CAD build for the part. Positions are in the model's coordinates, mm. A direction names the side the tool comes from. Give positions to 0.01 mm unless a question says otherwise; leave off trailing zeros. Order: outer loops, then holes, each group sorted by start corner. A loop starts at its lowest first (then second) coordinate and runs counter-clockwise, first axis right, second up. Notation, with made-up numbers: M -15.75,-7.5 L -10.75,-7.5 A13 cw -10.75,12.5 Z; hole C -1,71 d9. An arc over 180 degrees is marked long. Put each result on its own line as item: value. Start each with the question number.
1) Two-plate mould, pull along X, no slides. Class faces 1 (the face through (-26.03, 0.14, 1.61)), 2 (the face through (-0.296, 0.078, 15.872)), 3 (the face through (-19, 0, 0)): released by +X, released by -X, zero draft, split by the parting line, or undercut.
2) Cut at A-A (y = 0). Write the cut outline in (x, z) (3 decimals).
3) Drill centre lines: line 1 (Y direction, x = -22.86, z = 2.05) (3 decimals); line 2 (Z direction, x = 17.5, y = 2.5) (3 decimals); line 3 (X direction, y = -2.25, z = 9.5). Where is each one in solid material? Low to high. Write a range as [from, to].
4) Cut at C-C (z = 1.5). Write the cut outline in (x, y) (3 decimals), and give its area (3 significant figures).
5) Cut at B-B (x = -22.86). Write the cut outline in (y, z) (3 decimals).
6) Pin check, flat tips, straight feed: pin 1 (2 mm diameter, centred on y = 3, z = 14, fed in from -X); pin 2 (1.5 mm diameter, centred on y = 3, z = 5, fed in from +X). Stop position of each tip, or through.
7) Tool access for faces 4 (the face through (25.95, 1.31, 3.175)), 5 (the face through (19, 0, 0)), 6 (the face through (-26.1, 1.3, 3.175)): list every direction of +Z, -Z, +X, -X, +Y, -Y with a clear straight run to the whole face (end or side of a thin tool).
8) Cut at D-D (y = -4.75). Write the cut outline in (x, z) (3 decimals), and give its area (3 significant figures).
```python
from build123d import *

# Parameters (mm, degrees)
BOSS_EXTRUDE1_DEPTH = 5.5626
SKETCH2_R           = 3.175
CUT_EXTRUDE1_DEPTH  = 4.175


with BuildPart() as part:
    # Sketch1 → Boss-Extrude1 (new body, symmetric)
    with BuildSketch(Plane(origin=(0, 0, 0), x_dir=(1, 0, 0), z_dir=(0, 1, 0))):
        with BuildLine():
            Line((-12.7, 0), (-29.845, 0))
            Line((-29.845, 0), (-29.845, -3.175))
            Line((-29.845, -3.175), (-16.164461018, -3.175))
            ThreePointArc((-16.164461018, -3.175), (-15.693695846, -3.337813758), (-15.424104025, -3.756679389))
            ThreePointArc((-15.424104025, -3.756679389), (0, -15.875), (15.424104025, -3.756679389))
            ThreePointArc((15.424104025, -3.756679389), (15.693695846, -3.337813758), (16.164461018, -3.175))
            Line((16.164461018, -3.175), (29.845, -3.175))
            Line((29.845, -3.175), (29.845, 0))
            Line((29.845, 0), (12.7, 0))
            ThreePointArc((12.7, 0), (0, -12.7), (-12.7, 0))
        make_face()
    extrude(amount=BOSS_EXTRUDE1_DEPTH, both=True)

    # Sketch2 → Cut-Extrude1 (cut, through all)
    with BuildSketch(Plane.XY.offset(3.175)):
        with Locations((-22.86, 0)):
            Circle(SKETCH2_R)
        with Locations((22.86, 0)):
            Circle(SKETCH2_R)
    extrude(amount=-CUT_EXTRUDE1_DEPTH, mode=Mode.SUBTRACT)


solid = part.part
```
Solution:
1. face 1: undercut
1. face 2: split by the parting line
1. face 3: zero draft
2. outline: M -29.845,0 L -26.035,0 L -26.035,3.175 L -29.845,3.175 Z; M -19.685,0 L -12.7,0 A12.7 cw 12.7,0 L 19.685,0 L 19.685,3.175 L 16.164,3.175 A0.762 cw 15.424,3.757 A15.875 ccw -15.424,3.757 A0.762 cw -16.164,3.175 L -19.685,3.175 Z; M 26.035,0 L 29.845,0 L 29.845,3.175 L 26.035,3.175 Z
3. line 1: [-5.563, -3.175], [3.175, 5.563]
3. line 2: [0, 3.175]
3. line 3: [-12.72, -8.43], [8.43, 12.72]
4. outline: M -29.845,-5.563 L -12.611,-5.563 L -12.611,5.563 L -29.845,5.563 Z; M 12.611,-5.563 L 29.845,-5.563 L 29.845,5.563 L 12.611,5.563 Z; hole C -22.86,0 d6.35; hole C 22.86,0 d6.35
4. area: 320 mm²
5. outline: M -5.563,0 L -3.175,0 L -3.175,3.175 L -5.563,3.175 Z; M 3.175,0 L 5.563,0 L 5.563,3.175 L 3.175,3.175 Z
6. pin 1: x = -9.11
6. pin 2: x = 15.3
7. face 4: +Z, +X, +Y, -Y
7. face 5: -Z, +X, -X, +Y, -Y
7. face 6: +Z, -X, +Y, -Y
8. outline: M -29.845,0 L -12.7,0 A12.7 cw 12.7,0 L 29.845,0 L 29.845,3.175 L 16.164,3.175 A0.762 cw 15.424,3.757 A15.875 ccw -15.424,3.757 A0.762 cw -16.164,3.175 L -29.845,3.175 Z
8. area: 232 mm²
